from build123d import *

# Parameters (mm, degrees)
SKETCH1_W               = 8
SKETCH1_H               = 8
BOSS_EXTRUDE1_DEPTH     = 3
CUT_EXTRUDE1_DEPTH      = 12.704699911
CUT_EXTRUDE1_DEPTH_BACK = 12.704699911
CUT_EXTRUDE2_DEPTH      = 11
SKETCH4_R               = 1.75
CUT_EXTRUDE3_DEPTH      = 0.4
SKETCH5_W               = 8
SKETCH5_H               = 1
BOSS_EXTRUDE2_DEPTH     = 2
FILLET1_R               = 4
CUT_EXTRUDE4_DEPTH      = 0.4


with BuildPart() as part:
    # Sketch1 → Boss-Extrude1 (new body)
    with BuildSketch(Plane(origin=(0, 0, 0), x_dir=(1, 0, 0), z_dir=(0, 1, 0))):
        with Locations((4, 4)):
            Rectangle(SKETCH1_W, SKETCH1_H)
    extrude(amount=BOSS_EXTRUDE1_DEPTH)

    # Sketch2 → Cut-Extrude1 (cut, two sides: drawn at the far end of the back side and taken through both)
    with BuildSketch(Plane.XY.offset(-CUT_EXTRUDE1_DEPTH_BACK)):
        Polygon((0, 0), (0.6, 3), (0, 3), align=None)
        Polygon((8, 0), (7.4, 3), (8, 3), align=None)
    extrude(amount=CUT_EXTRUDE1_DEPTH + CUT_EXTRUDE1_DEPTH_BACK, mode=Mode.SUBTRACT)

    # Sketch3 → Cut-Extrude2 (cut)
    with BuildSketch(Plane(origin=(0, 0, 0), x_dir=(0, 0, -1), z_dir=(1, 0, 0))):
        Polygon((0, 0), (0.6, 3), (0, 3), align=None)
        Polygon((8, 3), (7.4, 3), (8, 0), align=None)
    extrude(amount=CUT_EXTRUDE2_DEPTH, mode=Mode.SUBTRACT)

    # Sketch4 → Cut-Extrude3 (cut)
    with BuildSketch(Plane.XZ):
        with Locations(Location((4, -3.75, 0), (0, 0, 270))):
            Circle(SKETCH4_R)
    extrude(amount=-CUT_EXTRUDE3_DEPTH, mode=Mode.SUBTRACT)

    # Sketch5 → Boss-Extrude2 (add)
    with BuildSketch(Plane.XZ):
        with Locations((4, -7.5)):
            Rectangle(SKETCH5_W, SKETCH5_H)
    extrude(amount=BOSS_EXTRUDE2_DEPTH)

    # Fillet1
    # the kernel refuses this fillet: 4 mm, written as the material it takes off along each edge
    with BuildSketch(Plane(origin=(8, -2, -16.660254038), x_dir=(0, 1, 0), z_dir=(0, 0, 1)), Plane(origin=(0, -2, 1.660254038), x_dir=(0, 1, 0), z_dir=(0, 0, -1))) as fillet1_piece_1:
        with BuildLine():
            CenterArc((4, 3.464101615), FILLET1_R, 180, 60)
            Line((0, 3.464101615), (-0.08, 3.464101615))
            Line((-0.08, 3.464101615), (-0.08, 0))
            Line((-0.08, 0), (0, -0.08))
            ThreePointArc((0, -0.08), (1, -0.08), (1.96, -0.069282032))
            Line((1.96, -0.069282032), (2, 0))
        make_face()
    extrude(amount=18.320508076, mode=Mode.SUBTRACT)

    # Sketch6 → Cut-Extrude4 (cut)
    with BuildSketch(Plane(origin=(0, 3, 0), x_dir=(1, 0, 0), z_dir=(0, 1, 0))):
        with BuildLine():
            Line((3.443331895, 5.130686034), (4.597178049, 5.130686034))
            Line((4.597178049, 5.130686034), (4.597178049, 4.291743727))
            add(Edge.make_bspline(
                [(4.597178049, 4.291743727), (4.596645702, 4.211170655), (4.595640561, 4.059038126), (4.578021597, 3.844434295), (4.553540207, 3.655975372), (4.51459395, 3.491238943), (4.462448704, 3.342468302), (4.388723742, 3.206338125), (4.298056147, 3.076066307), (4.187154731, 2.955594738), (4.059577941, 2.844170634), (3.913847481, 2.747275335), (3.753421756, 2.660946408), (3.638168327, 2.615497851), (3.579149203, 2.592224496)],
                knots=[0, 0, 0, 0, 1.347156832, 2.543608823, 3.599300285, 4.522475688, 5.370350604, 6.227678973, 7.103274953, 8.018757603, 8.959280198, 9.929437417, 10.939703653, 12, 12, 12, 12], degree=3))
            Line((3.579149203, 2.592224496), (3.366408818, 3.053762957))
            add(Edge.make_bspline(
                [(3.366408818, 3.053762957), (3.417874874, 3.07492834), (3.516080495, 3.11531534), (3.647721841, 3.193115232), (3.754216523, 3.284666717), (3.839841548, 3.388423011), (3.901059293, 3.510472084), (3.947065575, 3.648752862), (3.973734578, 3.806802537), (3.979016553, 3.918249261), (3.981793434, 3.976839881)],
                knots=[0, 0, 0, 0, 1.113959817, 2.125616841, 3.047494432, 3.914868512, 4.801521967, 5.765947312, 6.825496818, 8, 8, 8, 8], degree=3))
            Line((3.981793434, 3.976839881), (3.443331895, 3.976839881))
            Line((3.443331895, 3.976839881), (3.443331895, 5.130686034))
        make_face()
    extrude(amount=-CUT_EXTRUDE4_DEPTH, mode=Mode.SUBTRACT)


solid = part.part
Check sheet for the modelled part. Datum: model origin and axes. Units: mm. A direction names the side the tool comes from. Round coordinates to 2 decimals unless told otherwise and drop trailing zeros. Loops run counter-clockwise (first coordinate to the right, second up) from the corner with the lowest first, then second, coordinate; pieces in that order, holes last. Notation, with made-up numbers: (68.25, 49.25) -> (72.25, 49.25) arc R30 ccw to (72.25, 73.25) -> close; hole circle Ø11 at (-3, -8). An arc over 180 degrees is marked (long way). Put each result on its own line as item: value. Start each with the question number.
1. Gauge pin test, flat ends, axial feed: pin 1 (2 mm diameter, centred on x = 1, z = -4.5, fed in from -Y); pin 2 (1.6 mm diameter, centred on x = 6, y = -1, fed in from +Z); pin 3 (4 mm diameter, centred on x = 2, z = -5.5, fed in from -Y). Record the tip position at first contact, or that the pin passes through.
2. Section check C-C (z = -1.25). Enter the section's corners in (x, y).
3. Scan lines: probe 1 along X at (y, z) = (0.2, -3.75); probe 2 along Y at (x, z) = (4, -4.5); probe 3 along Y at (x, z) = (6.25, -1). Record each from-to range of solid material in increasing order.
4. Access from +Z, -Z, +X, -X, +Y, -Y to the whole of each face (thin tool, end or side, straight path). Record for faces 1 (the face through (4, -1, -7)), 2 (the face through (3.9, 1.5, -0.3)), 3 (the face through (2.94, 0.2, -2.36)).
5. Section check D-D (y = 2.2). Enter the section's corners in (x, z), plus the area to 3 significant figures.
6. Draft check along X on faces 4 (the face through (4, 2.6, -4.2)), 5 (the face through (7.7, 1.5, -4.1)), 6 (the face through (5, 3, -4)). Enter one of: +X half, -X half, draft (parallel to the pull), parting line (faces both ways), or undercut.
7. Section check B-B (x = 0.75). Enter the section's corners in (y, z), plus the area to 3 significant figures.
8. Section check A-A (y = 0.2). Enter the section's corners in (x, z), plus the area to 3 significant figures.
Findings:
1. pin 1: stops at y = 0
1. pin 2: stops at z = -7
1. pin 3: stops at y = -2
2. outline: (0, 0) -> (8, 0) -> (7.4, 3) -> (0.6, 3) -> close
3. probe 1: x = 0.04 to 2.25, 5.75 to 7.96
3. probe 2: y = 0.4 to 2.6
3. probe 3: y = 0 to 3
4. face 1: +Z, +X, -X, -Y
4. face 2: +Z, +X, -X, +Y
4. face 3: -Y
5. outline: (0.44, -7.56) -> (7.56, -7.56) -> (7.56, -0.44) -> (0.44, -0.44) -> close
5. area: 50.7 mm^2
6. face 4: undercut
6. face 5: +X half
6. face 6: draft
7. outline: (-0.94, -8) -> (0, -8) -> (3, -7.4) -> (3, -0.6) -> (0, 0) -> (0, -7) -> (-0.94, -7) -> close
7. area: 23.1 mm^2
8. outline: (0.04, -7.96) -> (7.96, -7.96) -> (7.96, -0.04) -> (0.04, -0.04) -> close; hole circle Ø3.5 at (4, -3.75)
8. area: 53.1 mm^2
